Geometry check sheet. Reference: the model listing, model coordinates, mm. A direction names the side the tool comes from. Give positions to 0.01 mm unless a question says otherwise; leave off trailing zeros. Write each loop counter-clockwise with the first axis right and the second up, starting at its lowest first coordinate (ties: lowest second). Pieces come first, ordered by that corner, then holes. Notation, with made-up numbers: (45, 69) -> (84, 69) arc R22 cw to (84, 95) -> close; hole circle Ø10 at (40.5, 44). An arc over 180 degrees is marked (long way). One line per item, written item: value.
from build123d import *

# Parameters (mm, degrees)
F0_W     = 80
F0_H     = 80
F0_W_2   = 74
F0_H_2   = 74
F1_DEPTH = 120
F3_DEPTH = 80.001
F4_R     = 3
F5_DEPTH = 25
F6_R     = 5


# Not quite as in the source:
# - a feature names something its author has since deleted; it is built from what else it names


with BuildPart() as f1:
    # F0 (on Front) → F1 (new body)
    with BuildSketch(Plane.XZ):
        Rectangle(F0_W, F0_H)
        Rectangle(F0_W_2, F0_H_2, mode=Mode.SUBTRACT)
    extrude(amount=F1_DEPTH)

    # F2 (on face) → F3 (cut, through all)
    with BuildSketch(Plane(origin=(-40, 0, 0), x_dir=(0, -1, 0), z_dir=(-1, 0, 0))):
        Polygon((120, -40), (120, 40), (105.8938415433, -40), align=None)
    extrude(amount=-F3_DEPTH, mode=Mode.SUBTRACT)

    # F4 (on face) → F5 (cut)
    with BuildSketch(Plane(origin=(0, 0, -40), x_dir=(1, 0, 0), z_dir=(0, 0, -1))):
        with Locations((0, 40)):
            Circle(F4_R)
    extrude(amount=-F5_DEPTH, mode=Mode.SUBTRACT)

    # F6
    f6_edges = [f1.edges().sort_by_distance(p)[0] for p in [
        (40, -60, 40),
        (40, -52.946921, -40),
        (-40, -60, 40),
        (-40, -52.946921, -40),
        (37, -59.73551, 37),
        (37, -53.211411, -37),
        (-37, -53.211411, -37),
        (-37, -59.73551, 37),
    ]]
    fillet(f6_edges, radius=F6_R)


solid = f1.part
1) Tool access check on faces 4 (the cylindrical face through (35, -54, -36)), 5 (the cylindrical face through (-39, -54, -38)), 6 (the cylindrical face through (0, -43, -39)). Record the directions out of +Z, -Z, +X, -X, +Y, -Y that give a thin tool (end or side, any length) a straight path to the whole face; none if there is none.
Verdict:
face 4: +Y, -Y
face 5: -Z, -X, +Y, -Y
face 6: -Z
2) Sectioned sample at B-B on x = 15. Record the cut outline in (y, z).
Verdict:
outline: (-120, 40) -> (-119.47, 37) -> (0, 37) -> (0, 40) -> close; (-106.42, -37) -> (-105.89, -40) -> (0, -40) -> (0, -37) -> close
3) Mould release check, pull along Z, two halves, no side actions. Record for faces 1 (the cylindrical face through (-39, -61, 38)), 2 (the cylindrical face through (-35, -61, 36)), 3 (the flat face through (-3, 0, -38)): released by +Z, released by -Z, zero draft, split by the parting line, or undercut.
Verdict:
face 1: released by +Z
face 2: undercut
face 3: zero draft
4) Scan lines: probe 1 along Z at (x, y) = (29, -72); probe 2 along X at (y, z) = (-40, -37.95). Record each from-to range of solid material in increasing order.
Verdict:
probe 1: -40 to -37, 37 to 40
probe 2: -39.04 to -3, 3 to 39.04
5) Sectioned sample at D-D on y = -14. Record the cut outline in (x, z), plus the area to 3 significant figures.
Verdict:
outline: (-40, -35) arc R5 ccw to (-35, -40) -> (35, -40) arc R5 ccw to (40, -35) -> (40, 35) arc R5 ccw to (35, 40) -> (-35, 40) arc R5 ccw to (-40, 35) -> close; hole (-37, -32) arc R5 ccw to (-32, -37) -> (32, -37) arc R5 ccw to (37, -32) -> (37, 32) arc R5 ccw to (32, 37) -> (-32, 37) arc R5 ccw to (-37, 32) -> close
area: 924 mm^2
6) Sectioned sample at C-C on z = -1.5. Record the cut outline in (x, y).
Verdict:
outline: (-40, -112.68) -> (-37, -112.68) -> (-37, 0) -> (-40, 0) -> close; (37, -112.68) -> (40, -112.68) -> (40, 0) -> (37, 0) -> close
7) Sectioned sample at A-A on x = 0. Record the cut outline in (y, z), plus the area to 3 significant figures.
Verdict:
outline: (-120, 40) -> (-119.47, 37) -> (0, 37) -> (0, 40) -> close; (-106.42, -37) -> (-105.89, -40) -> (-43, -40) -> (-43, -37) -> close; (-37, -40) -> (0, -40) -> (0, -37) -> (-37, -37) -> close
area: 660 mm^2
